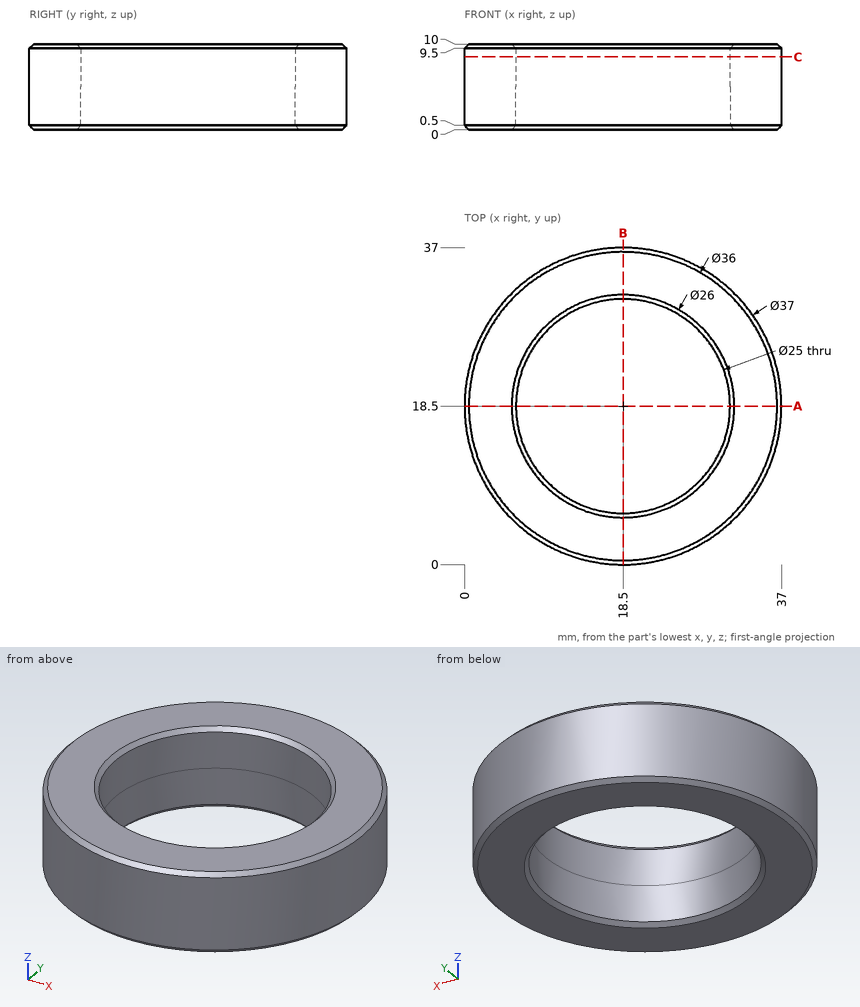
Check sheet for the drawn part. Datum: minimum x, y, z corner. Units: mm. Round coordinates to 2 decimals unless told otherwise and drop trailing zeros. Loops run counter-clockwise (first coordinate to the right, second up) from the corner with the lowest first, then second, coordinate; pieces in that order, holes last. Notation, with made-up numbers: M 81,76.5 L 117,76.5 A24 ccw 117,107.5 Z; hole C -12.5,47.25 d3. An arc over 180 degrees is marked long. One line per question, with ' | ' between items. Start each with the question number.
Item 1: Gauge pin test, flat ends, axial feed: pin 1 Ø2 at (y, z) = (7.5, 4) entering from +X; pin 2 Ø2 at (y, z) = (12, 4) entering from +X; pin 3 Ø15 at (x, y) = (18.5, 18.5) entering from +Z; pin 4 Ø8 at (x, y) = (24.5, 25) entering from +Z. Record the tip position at first contact, or that the pin passes through.
Item 2: Scan lines: probe 1 along Y at (x, z) = (18.5, 7.1); probe 2 along Y at (x, z) = (29, 2.25); probe 3 along X at (y, z) = (7, 4). Record each from-to range of solid material in increasing order.
Item 3: Section check A-A (y = 18.5). Record the boundary of the cut face in (x, z).
Item 4: Section check C-C (z = 8.5). Record the boundary of the cut face in (x, y).
Worked out:
1) pin 1: x = 34.06 | pin 2: x = 36.16 | pin 3: through | pin 4: z = 9.85
2) probe 1: 0 to 6, 31 to 37 | probe 2: 3.27 to 11.72, 25.28 to 33.73 | probe 3: 4.01 to 13.6, 23.4 to 32.99
3) outline: M 0,0.5 L 0.5,0 L 5.5,0 L 6,0.5 L 6,9.5 L 5.5,10 L 0.5,10 L 0,9.5 Z; M 31,0.5 L 31.5,0 L 36.5,0 L 37,0.5 L 37,9.5 L 36.5,10 L 31.5,10 L 31,9.5 Z
4) outline: C 18.5,18.5 d37; hole C 18.5,18.5 d25
